```python
from build123d import *

# Parameters (mm, degrees)
SKETCH1_W           = 20
SKETCH1_H           = 20
BOSS_EXTRUDE1_DEPTH = 10
SKETCH2_R           = 5
CUT_EXTRUDE1_DEPTH  = 3
SKETCH3_R           = 2
CUT_EXTRUDE2_DEPTH  = 3


with BuildPart() as part:
    # Sketch1 → Boss-Extrude1 (new body)
    with BuildSketch(Plane.XY):
        with Locations((10, 10)):
            Rectangle(SKETCH1_W, SKETCH1_H)
    extrude(amount=BOSS_EXTRUDE1_DEPTH)

    # Sketch2 → Cut-Extrude1 (cut)
    with BuildSketch(Plane.XY.offset(10)):
        with Locations((10, 10)):
            Circle(SKETCH2_R)
    extrude(amount=-CUT_EXTRUDE1_DEPTH, mode=Mode.SUBTRACT)

    # Sketch3 → Cut-Extrude2 (cut)
    with BuildSketch(Plane(origin=(0, 0, 0), x_dir=(-1, 0, 0), z_dir=(0, 0, -1))):
        with Locations((-13.9, 13.9)):
            Circle(SKETCH3_R)
        with Locations((-6.1, 13.9)):
            Circle(SKETCH3_R)
        with Locations((-13.9, 6.1)):
            Circle(SKETCH3_R)
        with Locations((-6.1, 6.1)):
            Circle(SKETCH3_R)
    extrude(amount=-CUT_EXTRUDE2_DEPTH, mode=Mode.SUBTRACT)


solid = part.part
```
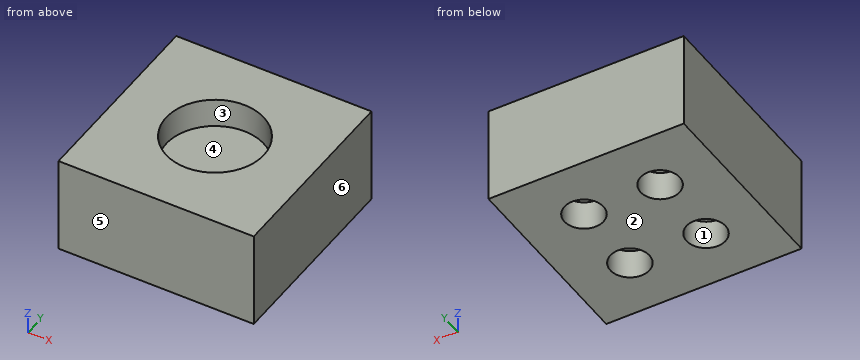
The listing builds one solid part. Answer for the finished solid, in the listing's coordinates (mm). Face numbers are marked on the shaded views. A direction names the side the tool comes from. Give positions to 0.01 mm unless a question says otherwise; leave off trailing zeros. Write each loop counter-clockwise with the first axis right and the second up, starting at its lowest first coordinate (ties: lowest second). Pieces come first, ordered by that corner, then holes. Notation, with made-up numbers: (22.5, 18) -> (52.5, 18) arc R22 cw to (52.5, 24) -> close; hole circle Ø6 at (-32, -5). An arc over 180 degrees is marked (long way). Write item = value, one per line. Start each with the question number.
1) The part is cut by section A-A, the plane z = 8.25. Determine the outline of the cut face in (x, y).
2) Which of the six approach directions +Z, -Z, +X, -X, +Y, -Y give full straight-line access (tool end or side, diameter ignored) to the marked faces 1, 2 and 3?
3) The part is cut by section C-C, the plane y = 13.9. Determine the outline of the cut face in (x, z), and give its area (3 significant figures).
4) Straight lines are drawn through the part: line 1 along Y through (x, z) = (6.1, 1.3); line 2 along Y through (x, z) = (5.25, 1.5); line 3 along Z through (x, y) = (11.25, 9). For each, find the intervals that lie inside material, in ascending order.
5) Determine the mould class of the marked faces 4, 5 and 6 for opening direction Y: +Y half, -Y half, draft (parallel to the pull), parting line (faces both ways), or undercut.
6) Each of these flat-tipped pins is pushed along its axis until it touches: pin 1 (1.2 mm diameter, centred on x = 14, y = 15, fed in from -Z); pin 2 (3 mm diameter, centred on x = 12, y = 11, fed in from +Z). Where does it stop, or does it pass through?
7) The part is cut by section B-B, the plane x = 10. Determine the outline of the cut face in (y, z).
Solutions:
q1.outline = (0, 0) -> (20, 0) -> (20, 20) -> (0, 20) -> close; hole circle Ø10 at (10, 10)
q2.face_1 = -Z
q2.face_2 = -Z, +X, -X, +Y, -Y
q2.face_3 = +Z
q3.outline = (0, 0) -> (4.1, 0) -> (4.1, 3) -> (8.1, 3) -> (8.1, 0) -> (11.9, 0) -> (11.9, 3) -> (15.9, 3) -> (15.9, 0) -> (20, 0) -> (20, 10) -> (13.13, 10) -> (13.13, 7) -> (6.87, 7) -> (6.87, 10) -> (0, 10) -> close
q3.area = 157 mm²
q4.line_1 = 0 to 4.1, 8.1 to 11.9, 15.9 to 20
q4.line_2 = 0 to 4.29, 7.91 to 12.09, 15.71 to 20
q4.line_3 = 0 to 7
q5.face_4 = undercut
q5.face_5 = -Y half
q5.face_6 = draft
q6.pin_1 = 3
q6.pin_2 = 7
q7.outline = (0, 0) -> (20, 0) -> (20, 10) -> (15, 10) -> (15, 7) -> (5, 7) -> (5, 10) -> (0, 10) -> close
